Geometry check sheet. Reference: drawing and pictorial views, mm from the part's lowest x, y, z. A direction names the side the tool comes from. Give positions to 0.01 mm unless a question says otherwise; leave off trailing zeros. Write each loop counter-clockwise with the first axis right and the second up, starting at its lowest first coordinate (ties: lowest second). Pieces come first, ordered by that corner, then holes. Notation, with made-up numbers: (23.5, 16.5) -> (48.5, 16.5) arc R18 ccw to (48.5, 31.5) -> close; hole circle Ø6 at (4, 3.25). An arc over 180 degrees is marked (long way). Return JSON: item names as keys, results as strings.
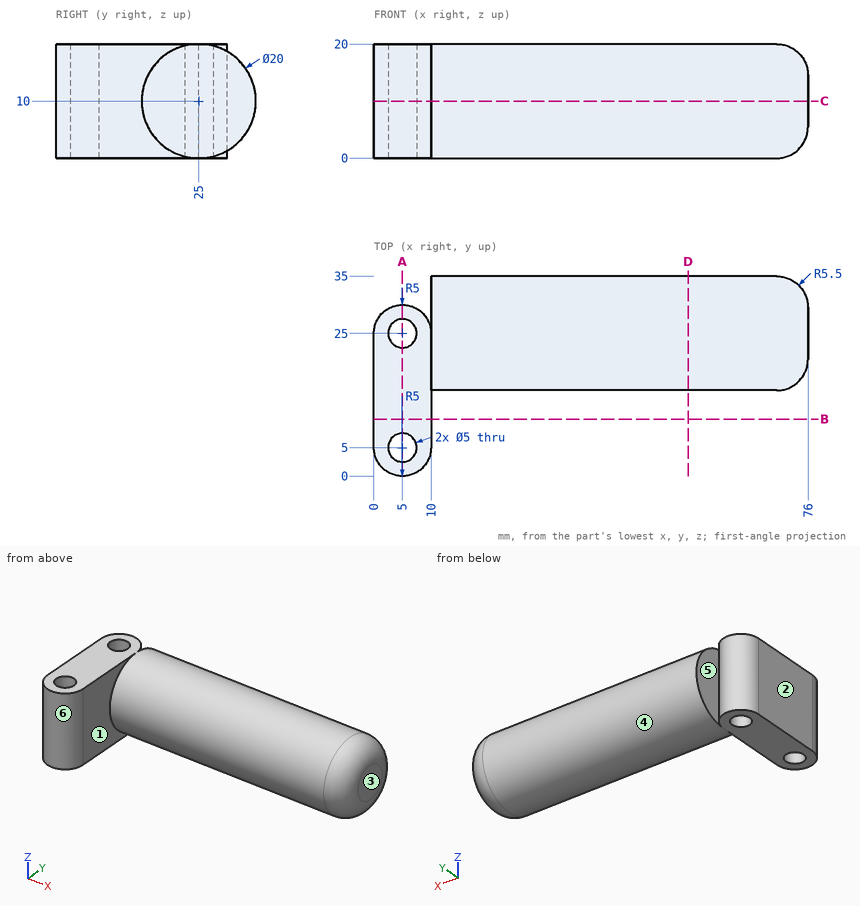
(1) Set-up check for the marked faces 1 and 2: record each of +Z, -Z, +X, -X, +Y, -Y from which the full face is reachable in a straight line by a thin tool's end or side.
Reply:
{"face 1": "+X, -Y", "face 2": "+Z, -Z, -X, +Y, -Y"}
(2) Release check for a two-part mould opening along X. For the marked faces 3, 4, 5 and 6 record: pulls with the +X half, pulls with the -X half, needs draft (parallel to the pull), parting line crosses it, or undercut.
Reply:
{"face 3": "pulls with the +X half", "face 4": "needs draft", "face 5": "undercut", "face 6": "parting line crosses it"}
(3) Cross-section at A-A on x = 5. Enter the section's corners in (y, z).
Reply:
{"outline": "(0, 0) -> (2.5, 0) -> (2.5, 20) -> (0, 20) -> close; (7.5, 0) -> (22.5, 0) -> (22.5, 20) -> (7.5, 20) -> close; (27.5, 0) -> (30, 0) -> (30, 20) -> (27.5, 20) -> close"}
(4) Cross-section at D-D on x = 55. Enter the section's corners in (y, z).
Reply:
{"outline": "circle Ø20 at (25, 10)"}
(5) Cross-section at C-C on z = 10. State how many separate pieces and enclosed holes the cut face has, then the cut area to 3 significant figures.
Reply:
{"separate pieces": "1", "enclosed holes": "2", "area": "1,550 mm^2"}
(6) Depth check by flat-ended pin: pin 1 Ø5 at (y, z) = (29.5, 7.5) entering from -X; pin 2 Ø4 at (x, y) = (48, 20) entering from -Z; pin 3 Ø12 at (x, z) = (13.5, 11) entering from -Y. Enter the tip coordinate at first touch or a pass-through.
Reply:
{"pin 1": "x = 0.42", "pin 2": "z = 0.46", "pin 3": "y = 0.67"}
(7) Thickness scan on L1, parallel to Y at x = 5, z = 6.25; L2, parallel to Y at x = 70, z = 9.75; L3, parallel to Z at x = 26, y = 24.5. Record the ranges inside material, lowest first.
Reply:
{"L1": "0 to 2.5, 7.5 to 22.5, 27.5 to 30", "L2": "15 to 35", "L3": "0.01 to 19.99"}
(8) Cross-section at B-B on y = 10. Enter the section's corners in (x, z), then the cut area to 3 significant figures.
Reply:
{"outline": "(0, 0) -> (10, 0) -> (10, 20) -> (0, 20) -> close", "area": "200 mm^2"}
